Verification items for the finished model (mm, model axes). Face numbers are marked on the shaded views. Give positions to 0.01 mm unless a question says otherwise; leave off trailing zeros. Order: outer loops, then holes, each group sorted by start corner. A loop starts at its lowest first (then second) coordinate and runs counter-clockwise, first axis right, second up. Notation, with made-up numbers: (44.25, -31.75) -> (73.25, -31.75) arc R30 cw to (73.25, -5.75) -> close; hole circle Ø6 at (47.5, -25.75). An arc over 180 degrees is marked (long way). One line per question, with ' | ' between items. Start each with the question number.
Q1. Mould release check, pull along X, two halves, no side actions. Record for the marked faces 1, 2 and 3: released by +X, released by -X, zero draft, split by the parting line, or undercut.
Q2. Material ranges on probe 1 along Y at (x, z) = (-5.5, 5.75); probe 2 along X at (y, z) = (1.5, 2.25); probe 3 along X at (y, z) = (10.5, 4.25), recorded low to high. Write a range as [from, to].
Q3. Section check B-B on x = -27. Record the cut outline in (y, z), plus the area to 3 significant figures.
Q4. Section check D-D on x = 21.5. Record the cut outline in (y, z), plus the area to 3 significant figures.
Q5. Section check A-A on z = 4.5. Give the number of separate pieces and of enclosed holes in the cut face, plus the area to 3 significant figures.
Q6. Go/stop test with flat-tipped pins: pin 1 (2 mm diameter, centred on x = 21, z = 1.5, fed in from -Y); pin 2 (3 mm diameter, centred on x = -28.5, z = 3.5, fed in from -Y); pin 3 (3 mm diameter, centred on x = -1, z = 2, fed in from -Y). Record where each tip stops, or that it passes through.
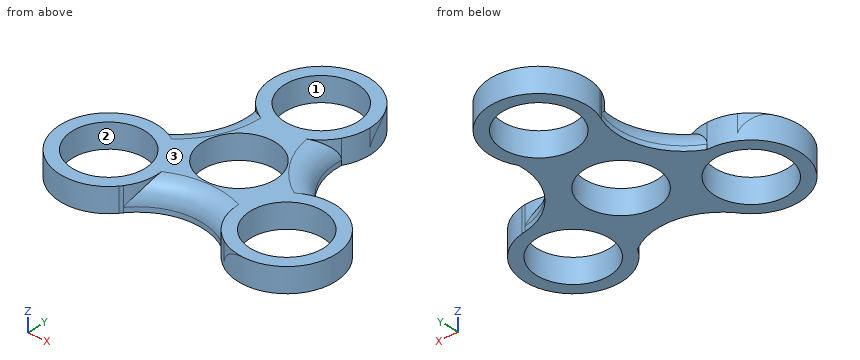
from build123d import *

# Parameters (mm, degrees)
F0_R         = 9.525
F1_DEPTH     = 6.35
F2_T4_ANGLE  = 171.8918539933
F2_S5_R      = 12.7
F2_T6_DEPTH  = 33
F2_S7_R      = 12.7
F2_T8_DEPTH  = 33
F2_T12_ANGLE = 171.8918539933
F2_S13_R     = 12.7
F2_T14_DEPTH = 34
F2_S15_R     = 12.7
F2_T16_DEPTH = 34
F2_T20_ANGLE = 171.8918539933
F2_S21_R     = 12.7
F2_T22_DEPTH = 33
F2_S23_R     = 12.7
F2_T24_DEPTH = 33


# Not quite as in the source:
# - a fillet or chamfer that OpenCascade refuses, or shapes differently, is made with other operations: its cross-section is extruded or revolved along the edge and cut away or added


with BuildPart() as f1:
    # F0 (on Top) → F1 (new body)
    with BuildSketch(Plane.XY):
        with BuildLine():
            ThreePointArc((-16.9151689036, 34.8937534074), (-16.926787396, 22.6379285555), (-25.2467054302, 13.6387985033))
            ThreePointArc((-25.2467054302, 13.6387985033), (-36.7990792752, -4.4780457484), (-15.4716495202, -7.0892001179))
            ThreePointArc((-15.4716495202, -7.0892001179), (-15.2019637006, -6.723178945), (-14.922490674, -6.3645750302))
            ThreePointArc((-14.922490674, -6.3645750302), (-4.3028257617, -0.2467245138), (7.6506084925, -2.9524198627))
            ThreePointArc((7.6506084925, -2.9524198627), (29.1164427734, -3.8986469606), (20.7140539132, 15.8770261894))
            ThreePointArc((20.7140539132, 15.8770261894), (20.2622273693, 15.9275703737), (19.8119307558, 15.9902991571))
            ThreePointArc((19.8119307558, 15.9902991571), (9.2038843359, 22.1282734926), (5.5703681159, 33.8330988937))
            ThreePointArc((5.5703681159, 33.8330988937), (-4.34309232, 52.8961702433), (-17.2681332147, 35.7316514628))
            ThreePointArc((-17.2681332147, 35.7316514628), (-17.0859924904, 35.3150861055), (-16.9151689036, 34.8937534074))
        make_face()
        with Locations((-25.31230589, 0.9389679304)):
            Circle(F0_R, mode=Mode.SUBTRACT)
        with Locations((-4.0085762739, 14.8398258448)):
            Circle(F0_R, mode=Mode.SUBTRACT)
        with Locations((18.6817846223, 3.3406837591)):
            Circle(F0_R, mode=Mode.SUBTRACT)
        with Locations((-5.3952075541, 40.2398258448)):
            Circle(F0_R, mode=Mode.SUBTRACT)
        with BuildLine():
            ThreePointArc((-14.922490674, -6.3645750302), (-15.2019637006, -6.723178945), (-15.4716495202, -7.0892001179))
            ThreePointArc((-15.4716495202, -7.0892001179), (-15.1905834316, -6.7318035089), (-14.922490674, -6.3645750302))
        make_face()
        with BuildLine():
            ThreePointArc((-17.2681332147, 35.7316514628), (-17.0991517164, 35.3095427854), (-16.9151689036, 34.8937534074))
            ThreePointArc((-16.9151689036, 34.8937534074), (-17.0859924904, 35.3150861055), (-17.2681332147, 35.7316514628))
        make_face()
        with BuildLine():
            ThreePointArc((19.8119307558, 15.9902991571), (20.2622273693, 15.9275703737), (20.7140539132, 15.8770261894))
            ThreePointArc((20.7140539132, 15.8770261894), (20.2640063262, 15.9417382578), (19.8119307558, 15.9902991571))
        make_face()
    extrude(amount=F1_DEPTH)

    # F2: fillet of radius 5.08 on 3 edges, made by hand


with BuildPart() as f2_tool2:
    # F2_s3 → F2_t4 (revolve)
    with BuildSketch(Plane(origin=(1.3219976545, -16.6427211425, 0), x_dir=(0, 0, 1), z_dir=(0.0791845597, -0.9968599729, 0))):
        with BuildLine():
            ThreePointArc((1.27, 19.9508919573), (4.8621024484, 21.4387895089), (6.35, 25.0308919573))
            Line((6.35, 25.0308919573), (6.35, 19.9508919573))
            Line((6.35, 19.9508919573), (1.27, 19.9508919573))
        make_face()
    revolve(axis=Axis((-1.7870715149, -16.8896868949, 6.35), (0, 0, -1)), revolution_arc=F2_T4_ANGLE)

    # F2_s5 → F2_t6 (cut, symmetric)
    with BuildSketch(Plane.XY.offset(2)):
        with Locations((-25.31230589, 0.9389679304)):
            Circle(F2_S5_R)
    extrude(amount=F2_T6_DEPTH, both=True, mode=Mode.SUBTRACT)

    # F2_s7 → F2_t8 (cut, symmetric)
    with BuildSketch(Plane.XY.offset(2)):
        with Locations((18.6817846223, 3.3406837591)):
            Circle(F2_S7_R)
    extrude(amount=F2_T8_DEPTH, both=True, mode=Mode.SUBTRACT)


with BuildPart() as f1_1:
    add(f1.part)

    # F2_t1: cut F2_tool2
    add(f2_tool2.part, mode=Mode.SUBTRACT)


with BuildPart() as f2_tool10:
    # F2_s11 → F2_t12 (revolve)
    with BuildSketch(Plane(origin=(30.4099792651, 20.9327995218, 0), x_dir=(0, 0, 1), z_dir=(0.8237137807, 0.5670058267, 0))):
        with BuildLine():
            ThreePointArc((1.27, 2.6333326422), (4.8621024484, 4.1212301938), (6.35, 7.7133326422))
            Line((6.35, 7.7133326422), (6.35, 2.6333326422))
            Line((6.35, 2.6333326422), (1.27, 2.6333326422))
        make_face()
    revolve(axis=Axis((22.3592354288, 32.6284617706, 6.35), (0, 0, -1)), revolution_arc=F2_T12_ANGLE)

    # F2_s13 → F2_t14 (cut, symmetric)
    with BuildSketch(Plane.XY.offset(2)):
        with Locations((18.6817846223, 3.3406837591)):
            Circle(F2_S13_R)
    extrude(amount=F2_T14_DEPTH, both=True, mode=Mode.SUBTRACT)

    # F2_s15 → F2_t16 (cut, symmetric)
    with BuildSketch(Plane.XY.offset(2)):
        with Locations((-5.3952075541, 40.2398258448)):
            Circle(F2_S15_R)
    extrude(amount=F2_T16_DEPTH, both=True, mode=Mode.SUBTRACT)


with BuildPart() as f1_2:
    add(f1_1.part)

    # F2_t9: cut F2_tool10
    add(f2_tool10.part, mode=Mode.SUBTRACT)


with BuildPart() as f2_tool18:
    # F2_s19 → F2_t20 (revolve)
    with BuildSketch(Plane(origin=(-37.7448413305, 17.9696603878, 0), x_dir=(0, 0, 1), z_dir=(-0.9028983404, 0.4298541461, 0))):
        with BuildLine():
            ThreePointArc((1.27, 28.8057387926), (4.8621024484, 30.2936363442), (6.35, 33.8857387926))
            Line((6.35, 33.8857387926), (6.35, 28.8057387926))
            Line((6.35, 28.8057387926), (1.27, 28.8057387926))
        make_face()
    revolve(axis=Axis((-32.5978927357, 28.7807026587, 6.35), (0, 0, -1)), revolution_arc=F2_T20_ANGLE)

    # F2_s21 → F2_t22 (cut, symmetric)
    with BuildSketch(Plane.XY.offset(2)):
        with Locations((-25.31230589, 0.9389679304)):
            Circle(F2_S21_R)
    extrude(amount=F2_T22_DEPTH, both=True, mode=Mode.SUBTRACT)

    # F2_s23 → F2_t24 (cut, symmetric)
    with BuildSketch(Plane.XY.offset(2)):
        with Locations((-5.3952075541, 40.2398258448)):
            Circle(F2_S23_R)
    extrude(amount=F2_T24_DEPTH, both=True, mode=Mode.SUBTRACT)


with BuildPart() as f1_3:
    add(f1_2.part)

    # F2_t17: cut F2_tool18
    add(f2_tool18.part, mode=Mode.SUBTRACT)


solid = f1_3.part
Filled in:
1) face 1: undercut | face 2: undercut | face 3: zero draft
2) probe 1: [2.27, 5.43], [24.25, 30.72], [49.76, 52.94] | probe 2: [-38, -34.82], [-15.8, 9.34], [28.03, 31.25] | probe 3: [-33.67, -12.49], [4.47, 12.4], [24.96, 29.17]
3) outline: (-11.65, 0) -> (-8.44, 0) -> (-8.44, 6.35) -> (-11.65, 6.35) -> close; (10.31, 0) -> (13.53, 0) -> (13.53, 6.35) -> (10.31, 6.35) -> close | area: 40.8 mm²
4) outline: (-9.04, 0) -> (-5.76, 0) -> (-5.76, 6.35) -> (-9.04, 6.35) -> close; (12.44, 0) -> (15.72, 0) -> (15.72, 6.35) -> (12.44, 6.35) -> close | area: 41.7 mm²
5) separate pieces: 1 | enclosed holes: 4 | area: 1,080 mm²
6) pin 1: y = -9.29 | pin 2: y = -11.65 | pin 3: y = -0.2
